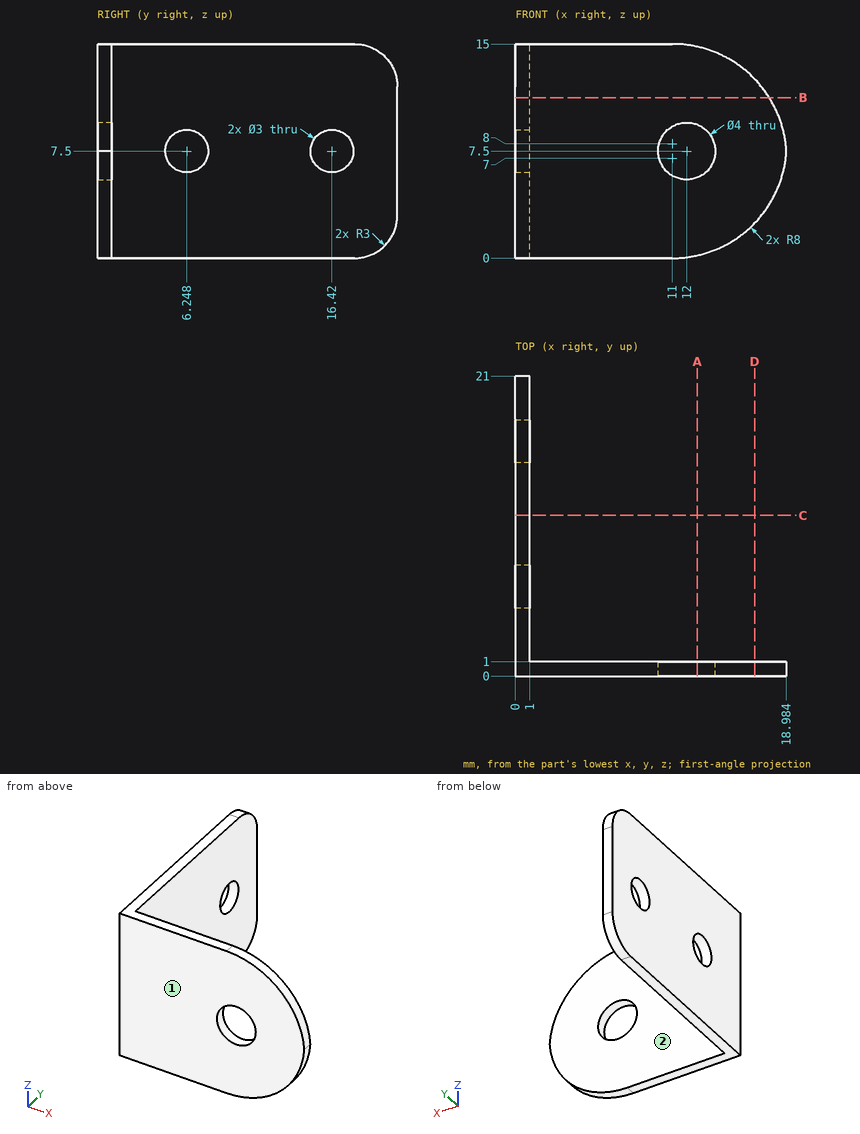
Verification items for this drawing (mm, ordinates from the low corner). A direction names the side the tool comes from. Give positions to 0.01 mm unless a question says otherwise; leave off trailing zeros. Loops run counter-clockwise (first coordinate to the right, second up) from the corner with the lowest first, then second, coordinate; pieces in that order, holes last. Notation, with made-up numbers: M -5.5,-18.5 L 19.5,-18.5 A24 cw 19.5,13.5 Z; hole C -6,-9.5 d3. An arc over 180 degrees is marked long. Answer as a JSON object with one key per item and string values. Group by question number.
Q1. Material ranges on line 1 along Y through (x, z) = (0.5, 7.5); line 2 along Y through (x, z) = (7, 8), recorded low to high. Write a range as [from, to].
Q2. Cross-section at C-C on y = 11.25. Record the cut outline in (x, z), then the cut area to 3 significant figures.
Q3. Go/stop test with flat-tipped pins: P1, Ø4.5, axis at x = 10.5, z = 6.5, coming from the +Y side; P2, Ø1.5, axis at y = 6, z = 1.5, coming from the +X side. Record where each tip stops, or that it passes through.
Q4. Cross-section at B-B on z = 11.25. Record the cut outline in (x, y).
Q5. Cross-section at A-A on x = 12.75. Record the cut outline in (y, z), then the cut area to 3 significant figures.
Q6. Access from +Z, -Z, +X, -X, +Y, -Y to the whole of each face (thin tool, end or side, straight path). Record for the marked faces 1 and 2.
Q7. Cross-section at D-D on x = 16.75. Record the cut outline in (y, z), then the cut area to 3 significant figures.
Evaluation:
{
 "1": {"line 1": "y = [0, 4.75], [7.75, 14.92], [17.92, 21]", "line 2": "y = [0, 1]"},
 "2": {"outline": "M 0,0 L 1,0 L 1,15 L 0,15 Z", "area": "15.0 mm2"},
 "3": {"P1": "stops at y = 1", "P2": "stops at x = 1"},
 "4": {"outline": "M 0,0 L 17.78,0 L 17.78,1 L 1,1 L 1,21 L 0,21 Z"},
 "5": {"outline": "M 0,0.19 L 1,0.19 L 1,5.65 L 0,5.65 Z; M 0,9.35 L 1,9.35 L 1,14.81 L 0,14.81 Z", "area": "10.9 mm2"},
 "6": {"face 1": "+Z, -Z, +X, -X, -Y", "face 2": "+Z, -Z, +X, +Y"},
 "7": {"outline": "M 0,2.44 L 1,2.44 L 1,12.56 L 0,12.56 Z", "area": "10.1 mm2"}
}
